CAD build for the part. Positions are in the model's coordinates, mm. Give positions to 0.01 mm unless a question says otherwise; leave off trailing zeros. Loops run counter-clockwise (first coordinate to the right, second up) from the corner with the lowest first, then second, coordinate; pieces in that order, holes last.
Autodesk Inventor part; units mm, degrees
ref_plane "YZ Plane" through (0, 0, 0) normal (1, 0, 0) x (0, 1, 0)
ref_plane "XZ Plane" through (0, 0, 0) normal (0, 1, 0) x (-1, 0, 0)
ref_plane "XY Plane" through (0, 0, 0) normal (0, 0, 1) x (1, 0, 0)
sketch "Sketch1" plane through (0, 0, 0) normal (0, 0, 1) x (1, 0, 0)
  line L0 (50, 15.95) -> (50, 19.05)
  line L1 (56.5, 15.95) -> (53.5, 15.95)
  line L2 (51, 15.95) -> (51, 15.95)
  line L3 (53.5, 14.45) -> (51, 14.45)
  line L4 (51, 20.55) -> (53.5, 20.55)
  line L5 (51, 14.45) -> (51, 15.95)
  line L6 (51, 19.05) -> (51, 20.55)
  line L7 (50, 19.05) -> (51, 19.05)
  line L8 (53.5, 19.05) -> (56.5, 19.05)
  line L9 (56.5, 15.95) -> (53.5, 15.95)
  line L10 (51, 15.95) -> (50, 15.95)
  line L11 (53.5, 20.55) -> (53.5, 19.05)
  line L12 (53.5, 15.95) -> (53.5, 14.45)
  line L13 (10, 15.95) -> (10, 19.05)
  line L14 (10, 19.05) -> (9, 19.05)
  line L15 (9, 14.45) -> (9, 15.95)
  line L16 (9, 19.05) -> (9, 20.55)
  line L17 (6, 20.55) -> (6, 19.05)
  line L18 (9, 20.55) -> (6, 20.55)
  line L19 (6, 15.95) -> (6, 14.45)
  line L20 (6, 19.05) -> (3, 19.05)
  line L21 (3, 15.95) -> (6, 15.95)
  line L22 (3, 15.95) -> (6, 15.95)
  line L23 (6, 14.45) -> (9, 14.45)
  line L24 (56.5, 19.05) -> (56.5, 41.9)
  line L25 (3, 15.95) -> (3, 9)
  line L26 (3, 9) -> (0, 9)
  line L27 (0, 9) -> (0, 0)
  line L28 (3, 19.05) -> (3, 41.9)
  line L29 (56.5, 41.9) -> (3, 41.9)
  line L30 (9, 15.95) -> (10, 15.95)
  line L31 (56.5, 15.95) -> (56.5, 9)
  line L32 (56.5, 9) -> (59.5, 9)
  line L33 (59.5, 9) -> (59.5, 0)
  line L34 (59.5, 0) -> (0, 0)
  circle A0 centre (45.6295, 23.05) radius 1.425
  circle A1 centre (18.6295, 23.05) radius 1.425
  circle A2 centre (18.6295, 33) radius 1.425
  circle A3 centre (45.6295, 33) radius 1.425
  circle A4 centre (45.6295, 23.05) radius 1.425
  circle A5 centre (45.6295, 33) radius 1.425
  circle A6 centre (18.6295, 33) radius 1.425
  circle A7 centre (18.6295, 23.05) radius 1.425
  line L35 (59.5, 9) -> (59.5, 17.5) construction
  line L36 (59.5, 17.5) -> (59.5, 15.95) construction
  line L37 (59.5, 15.95) -> (56.5, 15.95) construction
  dimension "d54" = 3.1
  dimension "d70" = 3.1
  dimension "d74" = 1.5
  dimension "d83" = 3
  dimension "d85" = 3.1
  dimension "d87" = 3
  dimension "d100" = 9
  dimension "d102" = 3.1
  dimension "d103" = 0
  dimension "d104" = 0
  dimension "d105" = 53.5
  dimension "d108" = 3
  dimension "d109" = 9
  dimension "d110" = 9
  dimension "d111" = 0
  dimension "d112" = 3
  dimension "d113" = 3
  dimension "d114" = 2.5
  dimension "d115" = 1
  dimension "d116" = 1
  dimension "d117" = 1.5
  dimension "d121" = 8.5
  dimension "d122" = 1.55
  dimension "d123" = 6.95
  dimension "d124" = 6.95
  dimension "d125" = 1
  dimension "d126" = 1
  dimension "d127" = 3
  dimension "d128" = 3
  dimension "d129" = 1.5
  dimension "d130" = 1.5
  dimension "d131" = 0
  dimension "d132" = 1.5
  dimension "d133" = 1.5
  dimension "d134" = 1.5
  dimension "d136" = 27
  dimension "d137" = 9.95
extrude "Extrusion1" add sketch "Sketch1" along normal blind 3
properties part number "Muñeca1"
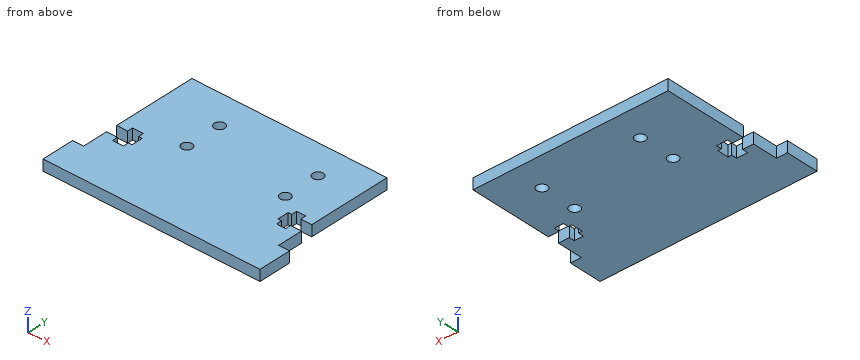
1. Drop flat-ended pins along their axis: pin 1 (1 mm diameter, centred on y = 13, z = 1.5, fed in from +X); pin 2 (1.5 mm diameter, centred on y = 18, z = 1.5, fed in from +X); pin 3 (1.6 mm diameter, centred on y = 20, z = 1.5, fed in from -X). Give the stop position or say it passes through.
Responses:
pin 1: stops at x = 56.5
pin 2: stops at x = 50
pin 3: stops at x = 3
2. Saw through at C-C, the plane y = 28. List the corners of the cut face in (x, z).
Responses:
outline: (3, 0) - (56.5, 0) - (56.5, 3) - (3, 3) - close
3. Saw through at A-A, the plane y = 23.05. List the corners of the cut face in (x, z).
Responses:
outline: (3, 0) - (17.2, 0) - (17.2, 3) - (3, 3) - close; (20.05, 0) - (44.2, 0) - (44.2, 3) - (20.05, 3) - close; (47.05, 0) - (56.5, 0) - (56.5, 3) - (47.05, 3) - close
4. Probe line 1 along X through (y, z) = (20, 1.05); line 2 along Y through (x, z) = (8, 2.75); line 3 along Y through (x, z) = (5, 1.75). List the from-to ranges inside material, lowest first.
Responses:
line 1: x = 3 to 6, 9 to 51, 53.5 to 56.5
line 2: y = 0 to 14.45, 20.55 to 41.9
line 3: y = 0 to 15.95, 19.05 to 41.9
5. Saw through at B-B, the plane z = 2.25. Count the separate pieces of the cut face and the enclosed holes in it, and give its area (3 significant figures).
Responses:
separate pieces: 1
enclosed holes: 4
area: 2,210 mm2
